from build123d import *

# Parameters (mm, degrees)
BOSS_EXTRUDE1_DEPTH  = 10
M4_CLEARANCE_HOLE1_D = 4.5


with BuildPart() as part:
    # Sketch1 → Boss-Extrude1 (new, symmetric)
    with BuildSketch(Plane(origin=(0, 0, 0), x_dir=(0, 0, -1), z_dir=(1, 0, 0))):
        with BuildLine():
            Line((-5.5, 0), (5.5, 0))
            Line((5.5, 0), (8, -4.330127019))
            ThreePointArc((8, -4.330127019), (7.816987298, -5.013139721), (7.133974596, -4.830127019))
            Line((7.133974596, -4.830127019), (4.922649731, -1))
            Line((4.922649731, -1), (-4.922649731, -1))
            Line((-4.922649731, -1), (-7.133974596, -4.830127019))
            ThreePointArc((-7.133974596, -4.830127019), (-7.816987298, -5.013139721), (-8, -4.330127019))
            Line((-8, -4.330127019), (-5.5, 0))
        make_face()
    extrude(amount=BOSS_EXTRUDE1_DEPTH, both=True)

    # M4 Clearance Hole1 (through all)
    with Locations(Plane(origin=(0, 0, 0), x_dir=(1, 0, 0), z_dir=(0, 1, 0))):
        with Locations((0, 0)):
            Hole(M4_CLEARANCE_HOLE1_D / 2)


solid = part.part
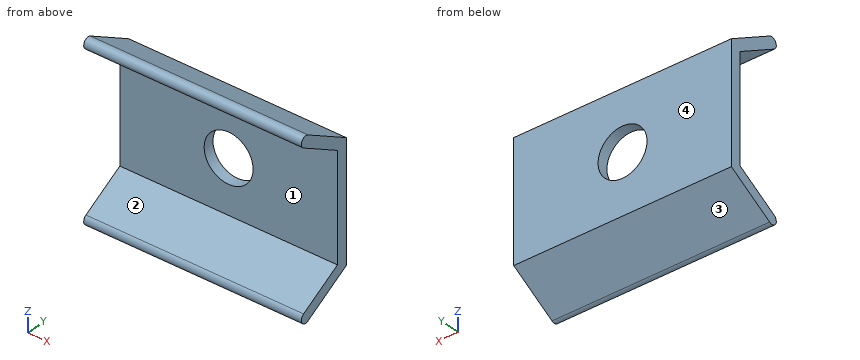
CAD build for the part. Positions are in the model's coordinates, mm. Face numbers are marked on the shaded views. Give positions to 0.01 mm unless a question says otherwise; leave off trailing zeros. Order: outer loops, then holes, each group sorted by start corner. A loop starts at its lowest first (then second) coordinate and runs counter-clockwise, first axis right, second up. Notation, with made-up numbers: (80.25, 27) - (101.25, 27) arc R17 cw to (101.25, 60) - close; hole circle Ø7 at (42, 19.25). An arc over 180 degrees is marked (long way). Answer in a Markdown table with one row per item.
1. Saw through at A-A, the plane z = 0. Give the cut face in (x, y), plus the area to 3 significant figures.
Data:
| item | result |
|---|---|
| outline | (-10, -1) - (-2.25, -1) - (-2.25, 0) - (-10, 0) - close; (2.25, -1) - (10, -1) - (10, 0) - (2.25, 0) - close |
| area | 15.5 mm² |
2. Saw through at D-D, the plane x = 6.25. Give the cut face in (y, z), plus the area to 3 significant figures.
Data:
| item | result |
|---|---|
| outline | (-4.83, -7.13) arc R0.5 ccw to (-4.33, -8) - (0, -5.5) - (0, 5.5) - (-4.33, 8) arc R0.5 ccw to (-4.83, 7.13) - (-1, 4.92) - (-1, -4.92) - close |
| area | 20.6 mm² |
3. Saw through at C-C, the plane y = -3.6. Give the cut face in (x, z), plus the area to 3 significant figures.
Data:
| item | result |
|---|---|
| outline | (-10, -7.58) - (10, -7.58) - (10, -6.42) - (-10, -6.42) - close; (-10, 6.42) - (10, 6.42) - (10, 7.58) - (-10, 7.58) - close |
| area | 46.2 mm² |
4. Pull direction Z, two halves, no side cores. Call the marked faces 1, 2, 3 and 4: pulls with the +Z half, pulls with the -Z half, needs draft (parallel to the pull), parting line crosses it, or undercut.
Data:
| item | result |
|---|---|
| face 1 | undercut |
| face 2 | undercut |
| face 3 | pulls with the -Z half |
| face 4 | needs draft |
5. Flat gauge pins, fed straight in: pin 1 (1 mm diameter, centred on x = -6, y = -1, fed in from +Z); pin 2 (1.5 mm diameter, centred on x = -6.5, y = -1, fed in from -Z); pin 3 (5 mm diameter, centred on x = -1.5, z = -4, fed in from -Y); pin 4 (2.5 mm diameter, centred on x = 0, z = 0, fed in from -Y). Where does each tip first touch, or does it go through?
Data:
| item | result |
|---|---|
| pin 1 | stops at z = 6.37 |
| pin 2 | stops at z = -6.51 |
| pin 3 | stops at y = -3.73 |
| pin 4 | passes through |
6. Saw through at B-B, the plane x = 0. Give the cut face in (y, z).
Data:
| item | result |
|---|---|
| outline | (-4.83, -7.13) arc R0.5 ccw to (-4.33, -8) - (0, -5.5) - (0, -2.25) - (-1, -2.25) - (-1, -4.92) - close; (-4.83, 7.13) - (-1, 4.92) - (-1, 2.25) - (0, 2.25) - (0, 5.5) - (-4.33, 8) arc R0.5 ccw to start |
7. Probe probe 1 along Y at (x, z) = (-6.5, 2); probe 2 along Z at (x, y) = (-8, -3.45); probe 3 along Z at (x, y) = (0, -0.45). List the from-to ranges inside material, lowest first. Write a range as [from, to].
Data:
| item | result |
|---|---|
| probe 1 | y = [-1, 0] |
| probe 2 | z = [-7.49, -6.34], [6.34, 7.49] |
| probe 3 | z = [-5.76, -2.25], [2.25, 5.76] |
